The listing builds one solid part. Answer for the finished solid, in the listing's coordinates (mm). Face numbers are marked on the shaded views. A direction names the side the tool comes from. Round coordinates to 2 decimals unless told otherwise and drop trailing zeros. Loops run counter-clockwise (first coordinate to the right, second up) from the corner with the lowest first, then second, coordinate; pieces in that order, holes last. Notation, with made-up numbers: M 42,17 L 89,17 A30 ccw 89,54 Z; hole C 6.5,-24.75 d3. An arc over 180 degrees is marked long. Put each result on its own line as item: value. Start each with the question number.
(1) Section C-C, the plane y = 27 is taken. Determine the outline of the cut face in (x, z).
(2) Determine the mould class of the marked faces 1, 2, 3 and 4 for opening direction Z: released by +Z, released by -Z, zero draft, split by the parting line, or undercut.
(3) Section A-A, the plane x = -9.5 is taken. Determine the outline of the cut face in (y, z), then the cut area to 3 significant figures.
(4) Section D-D, the plane z = 6 is taken. Determine the outline of the cut face in (x, y).
(5) Section B-B, the plane y = 14.5 is taken. Determine the outline of the cut face in (x, z) (3 decimals).
(6) Straight lines are drawn through the part: line 1 (X direction, y = 23, z = -48); line 2 (Z direction, x = -4, y = 31.5); line 3 (Y direction, x = -6.5, z = -13). For each, find the intervals that lie inside material, in ascending order.
(7) Flat-ended cylindrical pins translate along their axes: P1, Ø8, axis at y = 32.5, z = -20.5, coming from the -X side; P2, Ø5, axis at x = -7, z = -32, coming from the +Y side; P3, Ø12, axis at x = -13, z = 2, coming from the +Y side. Find the tip coordinate at first contact, or state that the pin passes through.
(8) Which of the six approach directions +Z, -Z, +X, -X, +Y, -Y give full straight-line access (tool end or side, diameter ignored) to the marked faces 5 and 6?
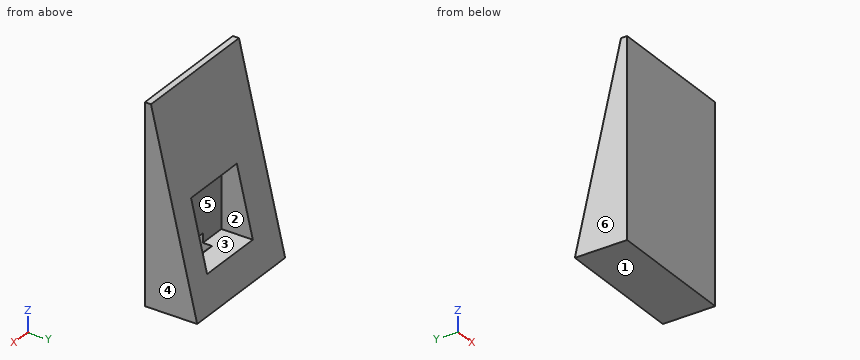
```python
from build123d import *

# Parameters (mm, degrees)
SKETCH1_W               = 100
SKETCH1_H               = 150
BOSS_EXTRUDE1_DEPTH     = 40
SKETCH3_W               = 52
SKETCH3_H               = 52
CUT_EXTRUDE2_DEPTH      = 30
CUT_EXTRUDE1_DEPTH      = 132.244047484
CUT_EXTRUDE5_DEPTH      = 10
CUT_EXTRUDE5_DEPTH_BACK = 5
SKETCH4_W               = 10
SKETCH4_H               = 10


with BuildPart() as part:
    # Sketch1 → Boss-Extrude1 (new body)
    with BuildSketch(Plane(origin=(0, 0, 0), x_dir=(1, 0, 0), z_dir=(0, 1, 0))):
        Rectangle(SKETCH1_W, SKETCH1_H)
    extrude(amount=BOSS_EXTRUDE1_DEPTH)

    # Sketch3 → Cut-Extrude2 (cut)
    with BuildSketch(Plane(origin=(0, 40, 0), x_dir=(1, 0, 0), z_dir=(0, 1, 0))):
        with Locations((4, 24)):
            Rectangle(SKETCH3_W, SKETCH3_H)
    extrude(amount=-CUT_EXTRUDE2_DEPTH, mode=Mode.SUBTRACT)

    # Sketch2 → Cut-Extrude1 (cut, through all)
    with BuildSketch(Plane(origin=(50, 0, 0), x_dir=(0, 0, -1), z_dir=(1, 0, 0))):
        Polygon((75, 40), (-95, 0), (-95, 40), align=None)
    extrude(amount=-CUT_EXTRUDE1_DEPTH, mode=Mode.SUBTRACT)

    # Sketch4 → Cut-Extrude5 (cut, two sides: drawn at the far end of the back side and taken through both)
    with BuildSketch(Plane(origin=(0, -20, -20), x_dir=(-1, 0, 0), z_dir=(0, 0.7071067811865477, 0.7071067811865475)).offset(-CUT_EXTRUDE5_DEPTH_BACK)):
        with Locations((-4, -42.426406871)):
            Rectangle(SKETCH4_W, SKETCH4_H)
    extrude(amount=CUT_EXTRUDE5_DEPTH + CUT_EXTRUDE5_DEPTH_BACK, mode=Mode.SUBTRACT)


solid = part.part
```
Recorded:
1. outline: M -50,-75 L 50,-75 L 50,-19.75 L 30,-19.75 L 30,-50 L -22,-50 L -22,-19.75 L -50,-19.75 Z
2. face 1: released by -Z
2. face 2: undercut
2. face 3: undercut
2. face 4: zero draft
3. outline: M 0,-75 L 40,-75 L 34.12,-50 L 10,-50 L 10,2 L 21.88,2 L 4.71,75 L 0,75 Z
3. area: 2,420 mm²
4. outline: M -50,0 L 50,0 L 50,20.94 L -50,20.94 Z
5. outline: M -50,-75 L 50,-75 L 50,33.375 L -50,33.375 Z; hole M -22,-50 L -1,-50 L -1,-52.571 L 9,-52.571 L 9,-50 L 30,-50 L 30,2 L -22,2 Z
6. line 1: x = -50 to -22, 30 to 50
6. line 2: z = -75 to -50
6. line 3: y = 0 to 10
7. P1: passes through
7. P2: stops at y = 10
7. P3: stops at y = 21.88
8. face 5: +Y
8. face 6: +Z, -Z, -X, +Y, -Y
